```python
from build123d import *

# Parameters (mm, degrees)
BASE_DEPTH                               = 9
BASE_DEPTH_BACK                          = 35
SKETCH1_W                                = 60
SKETCH1_H                                = 89
OUTSIDE_OF_BASE_R                        = 3
INSIDE_OF_BASE_T                         = -1.6
TOP_START                                = -44
TOP_FASTENING_BODY_DEPTH                 = 44
CBORE_FOR_M4_SHCS1_D                     = 4.8
CBORE_FOR_M4_SHCS1_CBORE_D               = 7.5
CBORE_FOR_M4_SHCS1_CBORE_DEPTH           = 4
TFB_START                                = -44
TFB_M_V_COPY_1_DEPTH                     = 44
TFB_M_V_COPY_2_D                         = 4.8
TFB_M_V_COPY_2_CBORE_D                   = 7.5
TFB_M_V_COPY_2_CBORE_DEPTH               = 4
SKETCH12_W                               = 8.4
SKETCH12_H                               = 3.5
MICROUSB_DEPTH                           = 1.6
F_3D_PRINTING_FOR_FASTENING_FEATURE_SIZE = 1.5
TFB_OUTER_R                              = 3
SKETCH28_W                               = 55
SKETCH28_H                               = 10
CUT_EXTRUDE1_DEPTH                       = 10


with BuildPart() as part:
    # Sketch1 → BASE (new, two sides: drawn at the far end of the back side and taken through both)
    with BuildSketch(Plane(origin=(0, 0, 0), x_dir=(1, 0, 0), z_dir=(0, 1, 0)).offset(-BASE_DEPTH_BACK)):
        Rectangle(SKETCH1_W, SKETCH1_H)
    extrude(amount=BASE_DEPTH + BASE_DEPTH_BACK)

    # OUTSIDE OF BASE
    outside_of_base_edges = [part.edges().sort_by_distance(p)[0] for p in [
        (30, -13, 44.5),
        (-30, -13, 44.5),
        (-30, -13, -44.5),
        (30, -13, -44.5),
    ]]
    fillet(outside_of_base_edges, radius=OUTSIDE_OF_BASE_R)

    # INSIDE OF BASE
    inside_of_base_openings = [part.faces().sort_by_distance(p)[0] for p in [
        (0, -35, 0),
    ]]
    offset(amount=INSIDE_OF_BASE_T, openings=inside_of_base_openings, kind=Kind.INTERSECTION)

    # Sketch22 → TOP FASTENING BODY (add)
    with BuildSketch(Plane.XZ.offset(35).offset(TOP_START)):
        with BuildLine():
            Line((-31.641355932, 49.085997649), (27, 44.5))
            Line((27, 44.5), (-27, 44.5))
            ThreePointArc((-27, 44.5), (-29.121320344, 43.621320344), (-30, 41.5))
            Line((-30, 41.5), (-30, 39.729546587))
            Line((-30, 39.729546587), (-32.358644068, 39.914002351))
            ThreePointArc((-32.358644068, 39.914002351), (-36.585997649, 44.858644068), (-31.641355932, 49.085997649))
        make_face()
    top_fastening_body = extrude(amount=TOP_FASTENING_BODY_DEPTH)

    # CBORE for M4 SHCS1 (through all)
    with Locations(Plane(origin=(0, 9, 0), x_dir=(1, 0, 0), z_dir=(0, 1, 0))):
        with Locations((-32, -44.5)):
            cbore_for_m4_shcs1 = CounterBoreHole(CBORE_FOR_M4_SHCS1_D / 2, CBORE_FOR_M4_SHCS1_CBORE_D / 2, CBORE_FOR_M4_SHCS1_CBORE_DEPTH)

    # TFB M H: TOP FASTENING BODY, CBORE for M4 SHCS1 across plane
    add(top_fastening_body.mirror(Plane(origin=(0, 0, 0), x_dir=(0, 0, 1), z_dir=(1, 0, 0))))
    add(cbore_for_m4_shcs1.mirror(Plane(origin=(0, 0, 0), x_dir=(0, 0, 1), z_dir=(1, 0, 0))), mode=Mode.SUBTRACT)

    # TFB M V: TOP FASTENING BODY, CBORE for M4 SHCS1 across plane
    add(top_fastening_body.mirror(Plane.XY))
    add(cbore_for_m4_shcs1.mirror(Plane.XY), mode=Mode.SUBTRACT)

    # TFB M V copy 1 sketch → TFB M V copy 1 (add)
    with BuildSketch(Plane(origin=(0, -35, 0), x_dir=(-1, 0, 0), z_dir=(0, -1, 0)).offset(TFB_START)):
        with BuildLine():
            Line((-31.641355932, 49.085997649), (27, 44.5))
            Line((27, 44.5), (-27, 44.5))
            ThreePointArc((-27, 44.5), (-29.121320344, 43.621320344), (-30, 41.5))
            Line((-30, 41.5), (-30, 39.729546587))
            Line((-30, 39.729546587), (-32.358644068, 39.914002351))
            ThreePointArc((-32.358644068, 39.914002351), (-36.585997649, 44.858644068), (-31.641355932, 49.085997649))
        make_face()
    extrude(amount=TFB_M_V_COPY_1_DEPTH)

    # TFB M V copy 2 (through all)
    with Locations(Plane(origin=(0, 9, 0), x_dir=(-1, 0, 0), z_dir=(0, 1, 0))):
        with Locations((-32, -44.5)):
            CounterBoreHole(TFB_M_V_COPY_2_D / 2, TFB_M_V_COPY_2_CBORE_D / 2, TFB_M_V_COPY_2_CBORE_DEPTH)

    # Sketch12 → MICROUSB (cut)
    with BuildSketch(Plane.ZY.offset(30)):
        with Locations((-31.9, -33.25)):
            Rectangle(SKETCH12_W, SKETCH12_H)
    extrude(amount=-MICROUSB_DEPTH, mode=Mode.SUBTRACT)

    # 3D PRINTING FOR FASTENING FEATURE
    # the kernel refuses this chamfer: 1.5 mm, written as the material it takes off along each edge
    with BuildSketch(Plane(origin=(32, 5, 44.5), x_dir=(1, 0, 0), z_dir=(0, 0, 1))) as f_3d_printing_for_fastening_feature_piece_1_section:
        Polygon((2.4 + F_3D_PRINTING_FOR_FASTENING_FEATURE_SIZE, 0), (2.4, -F_3D_PRINTING_FOR_FASTENING_FEATURE_SIZE), (2.4, 0), align=None)
    f_3d_printing_for_fastening_feature_piece_1 = revolve(axis=Axis((32, 5, 44.5), (0, 1, 0)), mode=Mode.PRIVATE)
    f_3d_printing_for_fastening_feature_piece_1 = f_3d_printing_for_fastening_feature_piece_1 & Plane(origin=(32, 4.173590616, 44.5), x_dir=(-1, 0, 0), z_dir=(0, 1, 0)) * Cylinder(3.75, 16, mode=Mode.PRIVATE)
    add(f_3d_printing_for_fastening_feature_piece_1, mode=Mode.SUBTRACT)
    with BuildSketch(Plane(origin=(32, 5, -44.5), x_dir=(1, 0, 0), z_dir=(0, 0, -1))) as f_3d_printing_for_fastening_feature_piece_2_section:
        Polygon((2.4 + F_3D_PRINTING_FOR_FASTENING_FEATURE_SIZE, 0), (2.4, F_3D_PRINTING_FOR_FASTENING_FEATURE_SIZE), (2.4, 0), align=None)
    f_3d_printing_for_fastening_feature_piece_2 = revolve(axis=Axis((32, 5, -44.5), (0, -1, 0)), mode=Mode.PRIVATE)
    f_3d_printing_for_fastening_feature_piece_2 = f_3d_printing_for_fastening_feature_piece_2 & Plane(origin=(32, 4.173590616, -44.5), x_dir=(-1, 0, 0), z_dir=(0, 1, 0)) * Cylinder(3.75, 16, mode=Mode.PRIVATE)
    add(f_3d_printing_for_fastening_feature_piece_2, mode=Mode.SUBTRACT)
    with BuildSketch(Plane(origin=(-32, 5, -44.5), x_dir=(-1, 0, 0), z_dir=(0, 0, -1))) as f_3d_printing_for_fastening_feature_piece_3_section:
        Polygon((2.4 + F_3D_PRINTING_FOR_FASTENING_FEATURE_SIZE, 0), (2.4, -F_3D_PRINTING_FOR_FASTENING_FEATURE_SIZE), (2.4, 0), align=None)
    f_3d_printing_for_fastening_feature_piece_3 = revolve(axis=Axis((-32, 5, -44.5), (0, 1, 0)), mode=Mode.PRIVATE)
    f_3d_printing_for_fastening_feature_piece_3 = f_3d_printing_for_fastening_feature_piece_3 & Plane(origin=(-32, 4.173590616, -44.5), x_dir=(1, 0, 0), z_dir=(0, 1, 0)) * Cylinder(3.75, 16, mode=Mode.PRIVATE)
    add(f_3d_printing_for_fastening_feature_piece_3, mode=Mode.SUBTRACT)
    with BuildSketch(Plane(origin=(-32, 5, 44.5), x_dir=(-1, 0, 0), z_dir=(0, 0, 1))) as f_3d_printing_for_fastening_feature_piece_4_section:
        Polygon((2.4 + F_3D_PRINTING_FOR_FASTENING_FEATURE_SIZE, 0), (2.4, F_3D_PRINTING_FOR_FASTENING_FEATURE_SIZE), (2.4, 0), align=None)
    f_3d_printing_for_fastening_feature_piece_4 = revolve(axis=Axis((-32, 5, 44.5), (0, -1, 0)), mode=Mode.PRIVATE)
    f_3d_printing_for_fastening_feature_piece_4 = f_3d_printing_for_fastening_feature_piece_4 & Plane(origin=(-32, 4.173590616, 44.5), x_dir=(1, 0, 0), z_dir=(0, 1, 0)) * Cylinder(3.75, 16, mode=Mode.PRIVATE)
    add(f_3d_printing_for_fastening_feature_piece_4, mode=Mode.SUBTRACT)

    # TFB OUTER
    tfb_outer_edges = [part.edges().sort_by_distance(p)[0] for p in [
        (30, -13, 39.729546587),
        (30, -13, -39.729546587),
        (-30, -13, -39.729546587),
        (-30, -13, 39.729546587),
    ]]
    fillet(tfb_outer_edges, radius=TFB_OUTER_R)

    # Sketch28 → Cut-Extrude1 (cut)
    with BuildSketch(Plane(origin=(30, 0, 0), x_dir=(0, 0, -1), z_dir=(1, 0, 0))):
        with Locations((5.877935747, -5)):
            Rectangle(SKETCH28_W, SKETCH28_H)
    extrude(amount=-CUT_EXTRUDE1_DEPTH, mode=Mode.SUBTRACT)


solid = part.part
```
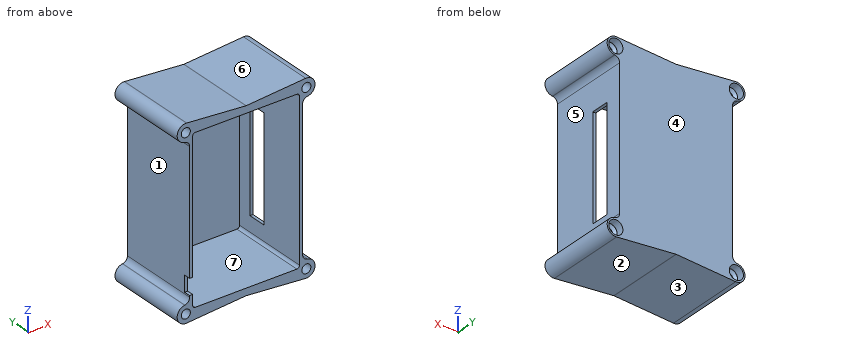
Source: CAD feature listing. Evaluate the final solid. Frame: model axes, mm. Face numbers are marked on the shaded views. A direction names the side the tool comes from. Coordinates: 2 decimals unless noted, no trailing zeros. Loops run counter-clockwise (first coordinate to the right, second up) from the corner with the lowest first, then second, coordinate; pieces in that order, holes last. Notation, with made-up numbers: M 62,47 L 78,47 A11 cw 78,63 Z; hole C -11.5,5.25 d6. An arc over 180 degrees is marked long. Use CSV: the item, a comma, the result in double quotes.
(1) Reachability of the marked faces 5, 6 and 7 from +Z, -Z, +X, -X, +Y, -Y: full face, straight path, thin tool, end or side. Return the list, or none.
Answers follow:
face 5,"+X, +Y, -Y"
face 6,"+Z, +Y, -Y"
face 7,"-Y"
(2) Cut plane B-B on z = -44.5. Return loops of the section in (x, y).
Answers follow:
outline,"M -36.6,-35 L -34.4,-35 L -34.4,3.5 L -35.75,4.85 L -35.75,9 L -36.6,9 Z; M -29.6,-35 L 29.6,-35 L 29.6,3.5 L 28.25,4.85 L 28.25,9 L -28.25,9 L -28.25,4.85 L -29.6,3.5 Z; M 34.4,-35 L 36.6,-35 L 36.6,9 L 35.75,9 L 35.75,4.85 L 34.4,3.5 Z"
(3) Cut plane A-A on z = 3. Return loops of the section in (x, y).
Answers follow:
outline,"M -30,-35 L -28.4,-35 L -28.4,7.4 L 28.4,7.4 L 28.4,0 L 30,0 L 30,9 L -30,9 Z; M 28.4,-35 L 30,-35 L 30,-10 L 28.4,-10 Z"
(4) Contact query for flat-ended pins moving along their axis: pin 1 (8.5 mm diameter, centred on x = -32, z = -44.5, fed in from +Y); pin 2 (2 mm diameter, centred on x = -22.5, y = -25, fed in from +Z); pin 3 (4.5 mm diameter, centred on x = -32, z = -44.5, fed in from -Y); pin 4 (1.8 mm diameter, centred on x = 29.5, y = -4.5, fed in from +Z). Output: stop coordinate, or through.
Answers follow:
pin 1,"y = 9"
pin 2,"z = 48.45"
pin 3,"through"
pin 4,"z = 48.99"
(5) Cut plane C-C on y = -12. Give the number of separate pieces and of enclosed holes in the cut face, and give its area (3 significant figures).
Answers follow:
separate pieces,"1"
enclosed holes,"5"
area,"1,000 mm²"
(6) Draft query along X for the marked faces 1, 2, 3 and 4. Return one class per face: pulls with the +X half, pulls with the -X half, needs draft (parallel to the pull), parting line crosses it, or undercut.
Answers follow:
face 1,"pulls with the -X half"
face 2,"undercut"
face 3,"undercut"
face 4,"needs draft"
(7) Line query: line 1 (X direction, y = -1.5, z = -42.5); line 2 (X direction, y = -22, z = -24); line 3 (Z direction, x = 33, y = -25.5). Output: solid intervals per line, ascending. Write a range as [from, to].
Answers follow:
line 1,"[-36.14, -33.33], [-30.67, -27.98], [27.98, 30.67], [33.33, 36.14]"
line 2,"[-30, -28.4], [28.4, 30]"
line 3,"[-48.99, -46.68], [-42.32, -40.01], [40.01, 42.32], [46.68, 48.99]"
(8) Cut plane D-D on x = -6. Return loops of the section in (y, z).
Answers follow:
outline,"M -35,-47.08 L 9,-47.08 L 9,47.08 L -35,47.08 L -35,42.9 L 7.4,42.9 L 7.4,-42.9 L -35,-42.9 Z"
